Can you work these out from the model? Positions are in its coordinate system, mm. A direction names the side the tool comes from. Give positions to 0.01 mm unless a question says otherwise; leave off trailing zeros. Write each loop counter-clockwise with the first axis right and the second up, starting at its lowest first coordinate (ties: lowest second). Pieces come first, ordered by that corner, then holes. Notation, with made-up numbers: (-25, -15.5) -> (4, -15.5) arc R31 cw to (4, 18.5) -> close; hole circle Ø2 at (49, 24). An arc over 180 degrees is marked (long way). One line per item, written item: value.
Autodesk Inventor part; units mm, degrees
ref_plane "YZ Plane" through (0, 0, 0) normal (1, 0, 0) x (0, 1, 0)
ref_plane "XZ Plane" through (0, 0, 0) normal (0, 1, 0) x (-1, 0, 0)
ref_plane "XY Plane" through (0, 0, 0) normal (0, 0, 1) x (1, 0, 0)
sketch "Sketch1" plane through (0, 0, 0) normal (0, 0, 1) x (1, 0, 0)
  arc A0 (0, 17.5133) -> (0, -17.5133) centre (0, 0) ccw
  arc A1 (194.9958, -17.5133) -> (194.9958, 17.5133) centre (194.9958, 0) ccw
  line L0 (0, 17.5133) -> (194.9958, 17.5133)
  line L1 (194.9958, -17.5133) -> (0, -17.5133)
  line L2 (194.9958, 20.0533) -> (0, 20.0533)
  arc A2 (0, 20.0533) -> (0, -20.0533) centre (0, 0) ccw
  line L3 (0, -20.0533) -> (194.9958, -20.0533)
  arc A3 (194.9958, -20.0533) -> (194.9958, 20.0533) centre (194.9958, 0) ccw
  dimension "d0" = 35.0266
  dimension "d1" = 194.9958
  dimension "d2" = 2.54
extrude "Extrusion1" add sketch "Sketch1" along normal blind 9
properties part number "INDX_022_SideBelt" material "Rubber"
1) I need wall thicknesses on L1, parallel to Y at x = 54.5, z = 7.5; L2, parallel to X at y = -1, z = 1.25; L3, parallel to X at y = 7.5, z = 4.5. Which ranges of each line are inside material? Lowest first, please.
Answer list:
L1: y = -20.05 to -17.51, 17.51 to 20.05
L2: x = -20.03 to -17.48, 212.48 to 215.02
L3: x = -18.6 to -15.83, 210.82 to 213.59
2) If we section it at A-A (x = 187.5): Write out the boundary of the cut face in (y, z), and give its area (3 significant figures).
Answer list:
outline: (-20.05, 0) -> (-17.51, 0) -> (-17.51, 9) -> (-20.05, 9) -> close; (17.51, 0) -> (20.05, 0) -> (20.05, 9) -> (17.51, 9) -> close
area: 45.7 mm^2
3) For faces 1 (the face through (97, 18, 0)), 2 (the face through (-17.51, -0.39, 4.44)), which set-ups out of +Z, -Z, +X, -X, +Y, -Y let a thin tool reach every point of the face, with its end or its side?
Answer list:
face 1: -Z, +X, -X, +Y, -Y
face 2: +Z, -Z
4) Will these pins go through, and if not, where does the flat tip stop? pin 1 (2 mm diameter, centred on y = -4.5, z = 2, fed in from -X); pin 2 (12 mm diameter, centred on x = 191.5, y = 9.5, fed in from +Z); pin 3 (4 mm diameter, centred on y = 7, z = 3.5, fed in from -X).
Answer list:
pin 1: stops at x = -19.75
pin 2: passes through
pin 3: stops at x = -19.42
5) We'd pull the mould along X, two halves only. Please class faces 3 (the face through (215.044, 0.441, 4.437)), 4 (the face through (96, 17.513, 4)), 5 (the face through (212.505, 0.385, 4.437)), 6 (the face through (-20.05, -0.44, 4.44)): released by +X, released by -X, zero draft, split by the parting line, or undercut.
Answer list:
face 3: released by +X
face 4: undercut
face 5: undercut
face 6: released by -X
6) If we section it at B-B (y = 0): Write out the boundary of the cut face in (x, z), and give its area (3 significant figures).
Answer list:
outline: (-20.05, 0) -> (-17.51, 0) -> (-17.51, 9) -> (-20.05, 9) -> close; (212.51, 0) -> (215.05, 0) -> (215.05, 9) -> (212.51, 9) -> close
area: 45.7 mm^2
